Autodesk Inventor part; units mm, degrees
ref_plane "YZ Plane" through (0, 0, 0) normal (1, 0, 0) x (0, 1, 0)
ref_plane "XZ Plane" through (0, 0, 0) normal (0, 1, 0) x (-1, 0, 0)
ref_plane "XY Plane" through (0, 0, 0) normal (0, 0, 1) x (1, 0, 0)
sketch "Skizze1" plane through (0, 0, 0) normal (0, 0, 1) x (1, 0, 0)
  circle A0 centre (0, 0) radius 33
  circle A1 centre (0, 0) radius 31
  dimension "d0" = 66
  dimension "d1" = 62
extrude "Extrusion1" add sketch "Skizze1" along normal mid plane 300
sketch "Skizze2" plane through (0, 0, 0) normal (0, 1, 0) x (-1, 0, 0)
  line L0 (-10, 169.5773) -> (-10, -169.8146) construction
  line L1 (-74.8376, 0) -> (82.6362, 0) construction
  line L2 (-10, 75) -> (-10, -75)
  line L3 (-33, -150) -> (-33, 150)
  line L4 (33, 150) -> (-33, 150)
  line L5 (-33, -150) -> (33, -150)
  spline S0 degree 2 poles (-10, 75) (-18.0478, 153.5197) (-72.8449, 128.3193) knots 0 0 0 1 1 1
  spline S1 degree 2 poles (-10, -75) (-17.6631, -153.0376) (-74.8376, -130) knots 0 0 0 1 1 1
  line L6 (33, -150) -> (-33, -150)
  line L7 (33, -150) -> (33, 150)
  line L8 (33, -150) -> (33, 150)
  line L9 (33, 150) -> (-33, 150)
  line L10 (-33, 150) -> (-33, 130)
  line L11 (-33, -150) -> (-33, 150)
  line L12 (33, -150) -> (-33, -150)
  point P0 (0, 0)
  point P1 (-33, -130)
  dimension "d4" = 10
  dimension "d5" = 150
  dimension "d6" = 20
  dimension "d7" = 20
extrude "Extrusion3" cut sketch "Skizze2" against normal mid plane 70 contours S0 L3 L4 L7 L5 S1 L2
properties part number "Segment_Deckel"
Verification items for the finished model (mm, model axes). Coordinates: 2 decimals unless noted, no trailing zeros. Loops run counter-clockwise (first coordinate to the right, second up) from the corner with the lowest first, then second, coordinate; pieces in that order, holes last. Notation, with made-up numbers: M -31,39 L -17,39 A21 ccw -17,49 Z; hole C 87,23 d5. An arc over 180 degrees is marked long. One line per item, written item: value.
1. Gauge pin test, flat ends, axial feed: P1, Ø10, axis at x = 23.5, z = 52.5, coming from the +Y side; P2, Ø6, axis at x = 26, y = -2, coming from the -Z side; P3, Ø6, axis at y = -7, z = -58.5, coming from the +X side; P4, Ø1.5, axis at x = 22.5, z = 89.5, coming from the -Y side. Record the tip position at first contact, or that the pin passes through.
Answers follow:
P1: y = 27.33
P2: through
P3: x = 32.76
P4: y = -24.82
2. Material ranges on line 1 along X through (y, z) = (10, 104.5); line 2 along Y through (x, z) = (23.75, -79.5); line 3 along Y through (x, z) = (23.5, 83.5), recorded low to high. Write a range as from..to.
Answers follow:
line 1: 29.34..31.45
line 2: -22.91..-19.92, 19.92..22.91
line 3: -23.17..-20.22, 20.22..23.17
3. Section check A-A on z = 37. Record the cut outline in (x, y).
Answers follow:
outline: M 10,-31.45 A33 ccw 10,31.45 L 10,29.34 A31 cw 10,-29.34 Z
